Source: three-view drawing plus pictorial views. Frame: mm from the lowest corner of the part. Coordinates: 2 decimals unless noted, no trailing zeros. Write each loop counter-clockwise with the first axis right and the second up, starting at its lowest first coordinate (ties: lowest second). Pieces come first, ordered by that corner, then holes. Notation, with made-up numbers: (16.5, -18) - (60.5, -18) arc R33 cw to (60.5, 13) - close; hole circle Ø5 at (-36, -26). An arc over 180 degrees is marked (long way). Put each result on its own line as item: value. Start each with the question number.
1. Pin query (flat end, axial travel): pin 1 (8 mm diameter, centred on x = 58, z = 10.5, fed in from +Y); pin 2 (5 mm diameter, centred on y = 21.5, z = 89.5, fed in from -X); pin 3 (5 mm diameter, centred on x = 75, y = 15, fed in from +Z). Return the tip coordinate at first contact, or that it passes through.
2. Cut plane D-D, the plane y = 4. Return loops of the section in (x, z).
3. Cut plane A-A, the plane z = 58. Return loops of the section in (x, y).
4. Pull-direction query (X, two-part tool) for the marked faces 1, 2 and 3; classes: released by +X, released by -X, zero draft, split by the parting line, or undercut.
5. Line query: line 1 (Y direction, x = 27, z = 54.5); line 2 (X direction, y = 24.75, z = 109); line 3 (X direction, y = 17.75, z = 66). Output: solid intervals per line, ascending.
6. Cut plane C-C, the plane x = 58. Return loops of the section in (y, z).
7. Cut plane B-B, the plane y = 14.25. Count the separate pieces of the cut face and the enclosed holes in it, and give its area (3 significant figures).
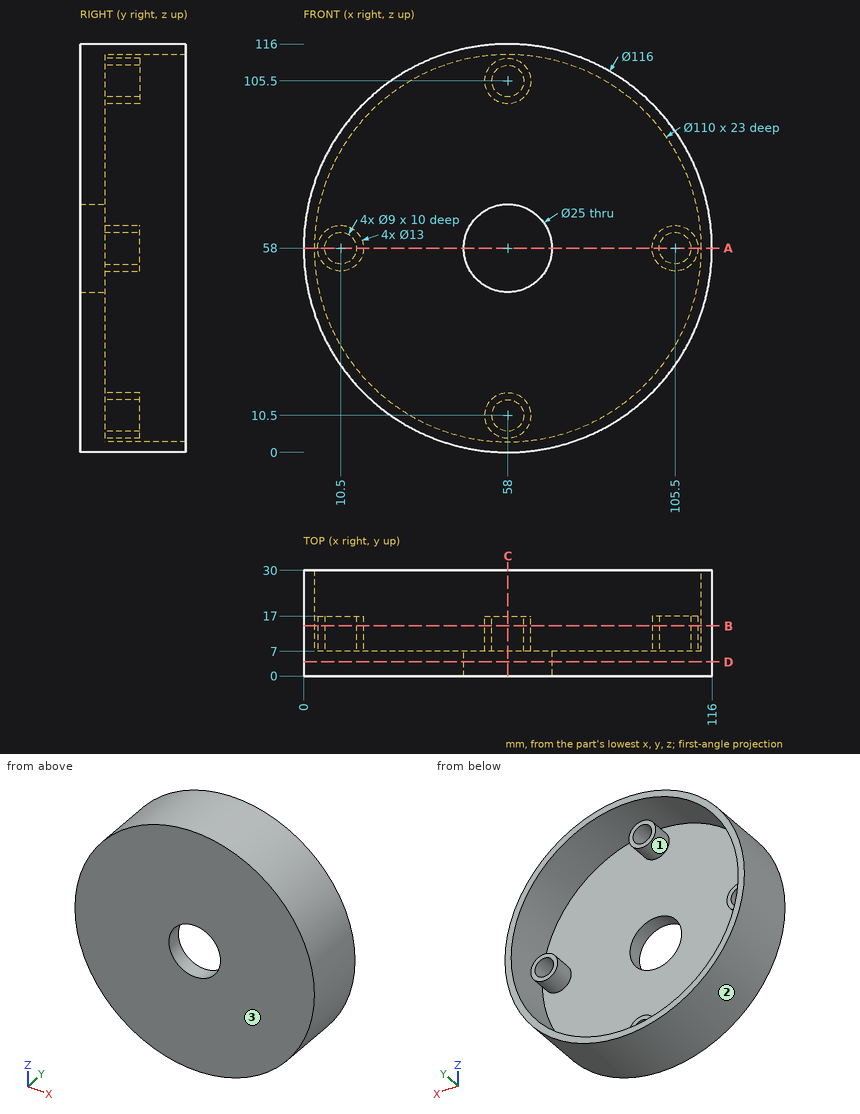
Report:
1. pin 1: stops at y = 7
1. pin 2: stops at x = 7.77
1. pin 3: stops at z = 114.16
2. outline: circle Ø116 at (58, 58); hole circle Ø25 at (58, 58)
3. outline: (0, 0) - (45.5, 0) - (45.5, 7) - (17, 7) - (17, 17) - (15, 17) - (15, 7) - (6, 7) - (6, 17) - (4, 17) - (4, 7) - (3, 7) - (3, 30) - (0, 30) - close; (70.5, 0) - (116, 0) - (116, 30) - (113, 30) - (113, 7) - (112, 7) - (112, 17) - (110, 17) - (110, 7) - (101, 7) - (101, 17) - (99, 17) - (99, 7) - (70.5, 7) - close
4. face 1: undercut
4. face 2: split by the parting line
4. face 3: zero draft
5. line 1: y = 0 to 7
5. line 2: x = 30.38 to 37.41, 78.59 to 85.62
5. line 3: x = 0.55 to 3.58, 112.42 to 115.45
6. outline: (0, 0) - (30, 0) - (30, 3) - (7, 3) - (7, 4) - (17, 4) - (17, 6) - (7, 6) - (7, 15) - (17, 15) - (17, 17) - (7, 17) - (7, 45.5) - (0, 45.5) - close; (0, 70.5) - (7, 70.5) - (7, 99) - (17, 99) - (17, 101) - (7, 101) - (7, 110) - (17, 110) - (17, 112) - (7, 112) - (7, 113) - (30, 113) - (30, 116) - (0, 116) - close
7. separate pieces: 5
7. enclosed holes: 5
7. area: 1,340 mm^2
